from build123d import *

# Parameters (mm, degrees)
F0_R     = 12.7
F1_DEPTH = 54.61
F2_DEPTH = 12.7
F3_DEPTH = 12.7
F4_R     = 5.08
F5_DEPTH = 19.05


with BuildPart() as f1:
    # F0 (on Front) → F1 (new body)
    with BuildSketch(Plane.XZ):
        with BuildLine():
            Line((-31.75, 0), (0, 0))
            Line((0, 0), (31.75, 0))
            Line((31.75, 0), (31.75, 12.7))
            Line((31.75, 12.7), (12.7, 12.7))
            Line((12.7, 12.7), (12.7, 21.59))
            Line((12.7, 21.59), (63.5, 21.59))
            Line((63.5, 21.59), (63.5, 34.29))
            Line((63.5, 34.29), (47.625, 34.29))
            Line((47.625, 34.29), (9.824759, 80.437615))
            ThreePointArc((9.824759, 80.437615), (5.435314, 83.868125), (0, 85.09))
            ThreePointArc((0, 85.09), (-5.435314, 83.868125), (-9.824759, 80.437615))
            Line((-9.824759, 80.437615), (-47.625, 34.29))
            Line((-47.625, 34.29), (-63.5, 34.29))
            Line((-63.5, 34.29), (-63.5, 21.59))
            Line((-63.5, 21.59), (-12.7, 21.59))
            Line((-12.7, 21.59), (-12.7, 12.7))
            Line((-12.7, 12.7), (-31.75, 12.7))
            Line((-31.75, 12.7), (-31.75, 0))
        make_face()
        with Locations((0, 59.69)):
            Circle(F0_R, mode=Mode.SUBTRACT)
    extrude(amount=F1_DEPTH)

    # F0 (on Front) → F2 (join)
    with BuildSketch(Plane.XZ):
        with Locations((0, 59.69)):
            Circle(F0_R)
    extrude(amount=F2_DEPTH)

    # F0 (on Front) → F3 (join)
    with BuildSketch(Plane.XZ):
        with BuildLine():
            Line((-63.5, 85.09), (-63.5, 34.29))
            Line((-63.5, 34.29), (-47.625, 34.29))
            Line((-47.625, 34.29), (-9.824759, 80.437615))
            ThreePointArc((-9.824759, 80.437615), (-5.435314, 83.868125), (0, 85.09))
            Line((0, 85.09), (-63.5, 85.09))
        make_face()
        with BuildLine():
            Line((47.625, 34.29), (63.5, 34.29))
            Line((63.5, 34.29), (63.5, 85.09))
            Line((63.5, 85.09), (0, 85.09))
            ThreePointArc((0, 85.09), (5.435314, 83.868125), (9.824759, 80.437615))
            Line((9.824759, 80.437615), (47.625, 34.29))
        make_face()
    extrude(amount=F3_DEPTH)

    # F4 (on face) → F5 (cut)
    with BuildSketch(Plane.XY.offset(85.09)):
        with Locations((0, -34.925)):
            Circle(F4_R)
    extrude(amount=-F5_DEPTH, mode=Mode.SUBTRACT)


solid = f1.part
Part model, mm, in its own coordinate system. A direction names the side the tool comes from. Coordinates: 2 decimals unless noted, no trailing zeros. Order: outer loops, then holes, each group sorted by start corner. A loop starts at its lowest first (then second) coordinate and runs counter-clockwise, first axis right, second up.
(1) Slice it at C-C, the plane z = 56.5. Write the cut outline in (x, y).
Check sheet entries:
outline: (-63.5, -12.7) - (-29.43, -12.7) - (-29.43, -54.61) - (-12.29, -54.61) - (-12.29, -12.7) - (12.29, -12.7) - (12.29, -54.61) - (29.43, -54.61) - (29.43, -12.7) - (63.5, -12.7) - (63.5, 0) - (-63.5, 0) - close
(2) Probe L1, parallel to Z at x = 0, y = -24; L2, parallel to Y at x = 44, z = 48; L3, parallel to X at y = -15, z = 59. List the from-to ranges inside material, lowest first.
Check sheet entries:
L1: z = 0 to 46.99, 72.39 to 85.09
L2: y = -12.7 to 0
L3: x = -27.38 to -12.68, 12.68 to 27.38
(3) Tool access for faces 1 (the face through (-46, -12.7, 66)), 2 (the face through (-31.75, -27, 6)), 3 (the face through (0, -12.7, 60)), 4 (the face through (12.7, -27, 17)), 5 (the face through (-22, -27, 12.7)): list every direction of +Z, -Z, +X, -X, +Y, -Y with a clear straight run to the whole face (end or side of a thin tool).
Check sheet entries:
face 1: +Z, -X, -Y
face 2: -Z, -X, +Y, -Y
face 3: -Y
face 4: +X, +Y, -Y
face 5: -X, +Y, -Y
(4) Slice it at D-D, the plane x = -22. Write the cut outline in (y, z), and give its area (3 significant figures).
Check sheet entries:
outline: (-54.61, 0) - (0, 0) - (0, 12.7) - (-54.61, 12.7) - close; (-54.61, 21.59) - (0, 21.59) - (0, 85.09) - (-12.7, 85.09) - (-12.7, 65.57) - (-54.61, 65.57) - close
area: 3,340 mm2
(5) Slice it at A-A, the plane y = -44. Write the cut outline in (x, z) (3 decimals), and give its area (3 significant figures).
Check sheet entries:
outline: (-63.5, 21.59) - (-12.7, 21.59) - (-12.7, 12.7) - (-31.75, 12.7) - (-31.75, 0) - (31.75, 0) - (31.75, 12.7) - (12.7, 12.7) - (12.7, 21.59) - (63.5, 21.59) - (63.5, 34.29) - (47.625, 34.29) - (9.825, 80.438) arc R12.7 ccw to (0, 85.09) arc R12.7 ccw to (-9.825, 80.438) - (-47.625, 34.29) - (-63.5, 34.29) - close; hole circle Ø25.4 at (0, 59.69)
area: 4,850 mm2
(6) Pin check, flat tips, straight feed: pin 1 Ø17.5 at (x, y) = (53, -27.5) entering from +Z; pin 2 Ø4 at (x, y) = (17, -18.5) entering from +Z; pin 3 Ø7 at (y, z) = (-21.5, 17.5) entering from -X. Stop position of each tip, or through.
Check sheet entries:
pin 1: stops at z = 38.41
pin 2: stops at z = 74.12
pin 3: stops at x = -12.7
(7) Slice it at B-B, the plane x = 29. Write the cut outline in (y, z).
Check sheet entries:
outline: (-54.61, 0) - (0, 0) - (0, 12.7) - (-54.61, 12.7) - close; (-54.61, 21.59) - (0, 21.59) - (0, 85.09) - (-12.7, 85.09) - (-12.7, 57.03) - (-54.61, 57.03) - close
(8) Pull direction Z, two halves, no side cores. Call faces 6 (the face through (38, -27, 21.59)), 7 (the face through (28.99, -33.36, 57.04)), 8 (the face through (63.5, -9, 39)): pulls with the +Z half, pulls with the -Z half, needs draft (parallel to the pull), parting line crosses it, or undercut.
Check sheet entries:
face 6: undercut
face 7: pulls with the +Z half
face 8: needs draft
